from build123d import *

# Parameters (mm, degrees)
F0_W      = 90
F0_H      = 50
F1_DEPTH  = 10
F2_W      = 90
F2_H      = 15
F3_DEPTH  = 40
F4_SIZE2  = 49.99999
F4_SIZE   = 19.99999
F5_SIZE2  = 19.99999
F5_SIZE   = 49.99999
F7_DEPTH  = 25
F8_DEPTH  = 15
F9_DEPTH  = 13
F10_DEPTH = 19
F11_R     = 4
F12_DEPTH = 40


# Not quite as in the source:
# - a fillet or chamfer is up to 0.001 mm smaller than in the source, because OpenCascade refuses the exact size


with BuildPart() as f1:
    # F0 (on Top) → F1 (new body)
    with BuildSketch(Plane.XY):
        with Locations((0.9217737243, 10.8652876893)):
            Rectangle(F0_W, F0_H)
    extrude(amount=F1_DEPTH)

    # F2 (on face) → F3 (join)
    with BuildSketch(Plane.XY.offset(10)):
        with Locations((0.9217737243, 18.3652876893)):
            Rectangle(F2_W, F2_H)
    extrude(amount=F3_DEPTH)

    # F4 (size 20 and 50 in the source; OpenCascade refuses exactly that, so slightly less here)
    f4_edges = [f1.edges().sort_by_distance(p)[0] for p in [
        (-44.078226, 18.365288, 50),
    ]]
    f4_side = f1.faces().sort_by_distance((0.921774, 18.365288, 50))[0]
    chamfer(f4_edges, length=F4_SIZE, length2=F4_SIZE2, reference=f4_side)

    # F5 (size 50 and 20 in the source; OpenCascade refuses exactly that, so slightly less here)
    f5_edges = [f1.edges().sort_by_distance(p)[0] for p in [
        (45.921774, 18.365288, 50),
    ]]
    f5_side = f1.faces().sort_by_distance((45.921774, 14.956197, 18.636364))[0]
    chamfer(f5_edges, length=F5_SIZE, length2=F5_SIZE2, reference=f5_side)

    # F6 (on face) → F7 (join)
    with BuildSketch(Plane.XZ.offset(-10.8652876893)):
        with BuildLine():
            Line((-17.3205080757, 50), (17.3205080757, 50))
            ThreePointArc((17.3205080757, 50), (0, 60), (-17.3205080757, 50))
        make_face()
        with BuildLine():
            Line((-18.3303027798, 48), (18.3303027798, 48))
            ThreePointArc((18.3303027798, 48), (17.8534332458, 49.0141511711), (17.3205080757, 50))
            Line((17.3205080757, 50), (-17.3205080757, 50))
            ThreePointArc((-17.3205080757, 50), (-17.8534332458, 49.0141511711), (-18.3303027798, 48))
        make_face()
        with BuildLine():
            ThreePointArc((6, 20.9212159717), (13.3669657075, 25.1230302893), (18.3303027798, 32))
            Line((18.3303027798, 32), (-18.3303027798, 32))
            ThreePointArc((-18.3303027798, 32), (-13.3669657075, 25.1230302893), (-6, 20.9212159717))
            ThreePointArc((-6, 20.9212159717), (0, 20), (6, 20.9212159717))
        make_face()
    extrude(amount=F7_DEPTH)

    # F8 (add): a face of the model
    f8_faces = [f1.faces().sort_by_distance(p)[0] for p in [
        (0, 10.8652876893, 54.100403238),
    ]]
    extrude(f8_faces, amount=F8_DEPTH)

    # F6 (on face) → F9 (join)
    with BuildSketch(Plane.XZ.offset(-10.8652876893)):
        with BuildLine():
            ThreePointArc((18.3303027798, 32), (19.5781262586, 35.9138071262), (20, 40))
            ThreePointArc((20, 40), (19.5781262586, 44.0861928738), (18.3303027798, 48))
            Line((18.3303027798, 48), (-18.3303027798, 48))
            ThreePointArc((-18.3303027798, 48), (-20, 40), (-18.3303027798, 32))
            Line((-18.3303027798, 32), (18.3303027798, 32))
        make_face()
    extrude(amount=F9_DEPTH)

    # F6 (on face) → F10 (join)
    with BuildSketch(Plane.XZ.offset(-10.8652876893)):
        with BuildLine():
            Line((6, 10), (6, 20.9212159717))
            ThreePointArc((6, 20.9212159717), (0, 20), (-6, 20.9212159717))
            Line((-6, 20.9212159717), (-6, 10))
            Line((-6, 10), (6, 10))
        make_face()
    extrude(amount=F10_DEPTH)

    # F11 (on face) → F12 (cut)
    with BuildSketch(Plane.XZ.offset(2.1347123107)):
        with Locations((0, 40)):
            Circle(F11_R)
    extrude(amount=-F12_DEPTH, mode=Mode.SUBTRACT)


solid = f1.part
Geometry check sheet. Reference: the model listing, model coordinates, mm. A direction names the side the tool comes from. Coordinates: 2 decimals unless noted, no trailing zeros. Order: outer loops, then holes, each group sorted by start corner. A loop starts at its lowest first (then second) coordinate and runs counter-clockwise, first axis right, second up. Notation, with made-up numbers: (86.5, -36) - (102.5, -36) arc R20 cw to (102.5, -18) - close; hole circle Ø8 at (63, 19). An arc over 180 degrees is marked (long way). Answer in a Markdown table with one row per item. Add a question column.
1) Material ranges on line 1 along Z through (x, y) = (0, 14); line 2 along Z through (x, y) = (12, -9); line 3 along Y through (x, z) = (6, 38), recorded low to high. Write a range as [from, to].
2) Cross-section at C-C, the plane z = 40. Record the cut outline in (x, y), then the cut area to 3 significant figures.
3) Set-up check for faces 4 (the flat face through (-21, 18, 50)), 5 (the flat face through (0, 25.865, 29)), 6 (the flat face through (0, -8, 48)), 7 (the cylindrical face through (-3.836, 6.145, 59.629)), 8 (the flat face through (-23, 10.865, 21)): record each of +Z, -Z, +X, -X, +Y, -Y from which the full face is reachable in a straight line by a thin tool's end or side.
4) Cross-section at D-D, the plane z = 26.5. Record the cut outline in (x, y), then the cut area to 3 significant figures.
5) Release check for a two-part mould opening along Z. For faces 1 (the flat face through (0, -14.135, 5)), 2 (the flat face through (22, 18, 50)), 3 (the flat face through (4.2, -2.135, 40.1)) record: +Z half, -Z half, draft (parallel to the pull), parting line (faces both ways), or undercut.
6) Cross-section at B-B, the plane x = 0. Record the cut outline in (y, z).
7) Gauge pin test, flat ends, axial feed: P1, Ø12, axis at y = -1, z = 15.5, coming from the -X side; P2, Ø1, axis at y = 26, z = 21, coming from the +X side; P3, Ø2, axis at x = -20.5, y = 15, coming from the +Z side; P4, Ø12, axis at x = -5, y = 10, coming from the -Z side. Record the tip position at first contact, or that the pin passes through.
Check result:
| question | item | result |
|---|---|---|
| 1 | line 1 | z = [0, 36], [44, 60] |
| 1 | line 2 | z = [0, 10], [24, 32], [48, 56] |
| 1 | line 3 | y = [-2.13, 25.87] |
| 2 | outline | (-28.08, 10.87) - (-20, 10.87) - (-20, -2.13) - (-4, -2.13) - (-4, 25.87) - (-28.08, 25.87) - close; (4, -2.13) - (20, -2.13) - (20, 10.87) - (29.92, 10.87) - (29.92, 25.87) - (4, 25.87) - close |
| 2 | area | 1,170 mm² |
| 3 | face 4 | +Z, -X, +Y, -Y |
| 3 | face 5 | +Z, +X, -X, +Y |
| 3 | face 6 | +X, -X, -Y |
| 3 | face 7 | -Y |
| 3 | face 8 | -X, -Y |
| 4 | outline | (-33.48, 10.87) - (-14.76, 10.87) - (-14.76, -14.13) - (14.76, -14.13) - (14.76, 10.87) - (35.32, 10.87) - (35.32, 25.87) - (-33.48, 25.87) - close |
| 4 | area | 1,770 mm² |
| 5 | face 1 | draft |
| 5 | face 2 | +Z half |
| 5 | face 3 | undercut |
| 6 | outline | (-14.13, 0) - (35.87, 0) - (35.87, 10) - (25.87, 10) - (25.87, 36) - (-2.13, 36) - (-2.13, 32) - (-14.13, 32) - (-14.13, 20) - (-8.13, 20) - (-8.13, 10) - (-14.13, 10) - close; (-14.13, 48) - (-2.13, 48) - (-2.13, 44) - (25.87, 44) - (25.87, 60) - (-14.13, 60) - close |
| 7 | P1 | stops at x = -40.28 |
| 7 | P2 | stops at x = 37.71 |
| 7 | P3 | stops at z = 50 |
| 7 | P4 | stops at z = 0 |
